Work out the finished part from the listing and answer in its coordinate system (mm). Face numbers are marked on the shaded views. A direction names the side the tool comes from. Coordinates: 2 decimals unless noted, no trailing zeros. Order: outer loops, then holes, each group sorted by start corner. A loop starts at its lowest first (then second) coordinate and runs counter-clockwise, first axis right, second up. Notation, with made-up numbers: M -21,19.5 L 17,19.5 A17 ccw 17,36.5 Z; hole C 62,43 d2. An arc over 180 degrees is marked long. Use a Markdown table: item, result.
from build123d import *

# Parameters (mm, degrees)
BOSS_EXTRUDE1_DEPTH     = 76.2
CHAMFER1_SIZE           = 16.51
CHAMFER2_SIZE           = 1
CUT_EXTRUDE1_DEPTH      = 3.425
SKETCH5_R               = 1.905
CUT_EXTRUDE2_DEPTH      = 114.174020707
CUT_EXTRUDE3_DEPTH      = 118.371627589
CUT_EXTRUDE3_DEPTH_BACK = 12.7
SKETCH6_R               = 6.35
SKETCH5_3_R             = 3.81
CUT_EXTRUDE4_DEPTH      = 12.7


with BuildPart() as part:
    # Sketch1 → Boss-Extrude1 (new body)
    with BuildSketch(Plane(origin=(0, 0, 0), x_dir=(1, 0, 0), z_dir=(0, 1, 0))):
        Polygon((-25.4, 47.146344636), (25.4, 47.146344636), (72.546344636, 0), (25.4, -47.146344636), (-25.4, -47.146344636), (-72.546344636, 0), align=None)
    extrude(amount=BOSS_EXTRUDE1_DEPTH)

    # SurfaceCut1
    split(bisect_by=Plane(origin=(0, 10.036699622, 10.036699622), x_dir=(-1, 0, 0), z_dir=(0, 0.7071067811865464, 0.7071067811865488)), keep=Keep.TOP)

    # SurfaceCut2
    split(bisect_by=Plane(origin=(0, 10.036699622, -10.036699622), x_dir=(1, 0, 0), z_dir=(0, 0.7071067811865464, -0.7071067811865488)), keep=Keep.TOP)

    # SurfaceCut3
    split(bisect_by=Plane(origin=(0, 50.8, 0), x_dir=(1, 0, 0), z_dir=(0, 1, 0)), keep=Keep.TOP)

    # Chamfer1
    chamfer1_edges = [part.edges().sort_by_distance(p)[0] for p in [
        (-57.183044257, 50.8, 15.363300378),
        (-57.183044257, 50.8, -15.363300378),
        (57.183044257, 50.8, 15.363300378),
        (57.183044257, 50.8, -15.363300378),
    ]]
    chamfer(chamfer1_edges, length=CHAMFER1_SIZE)

    # Chamfer2
    chamfer2_edges = [part.edges().sort_by_distance(p)[0] for p in [
        (72.546344636, 71.755, 0),
        (-72.546344636, 71.755, 0),
        (0, 76.2, 47.146344636),
        (48.973172318, 76.2, 23.573172318),
        (48.973172318, 76.2, -23.573172318),
        (0, 76.2, -47.146344636),
        (-48.973172318, 76.2, -23.573172318),
        (-48.973172318, 76.2, 23.573172318),
    ]]
    chamfer(chamfer2_edges, length=CHAMFER2_SIZE)

    # Sketch2 → Cut-Extrude1 (cut)
    with BuildSketch(Plane(origin=(0, 76.2, 0), x_dir=(1, 0, 0), z_dir=(0, 1, 0))):
        Polygon((-23.68275885, 45.681605271), (-69.36436412, 0), (-23.682753383, -45.681610738), align=None)
        Polygon((69.36436412, 0), (23.682756199, 45.681607921), (23.682745222, -45.681618898), align=None)
    extrude(amount=-CUT_EXTRUDE1_DEPTH, mode=Mode.SUBTRACT)

    # Sketch5 → Cut-Extrude2 (cut, through all)
    with BuildSketch(Plane(origin=(0, 10.036699622, -10.036699622), x_dir=(1, 0, 0), z_dir=(0, 0.7071067811865464, -0.7071067811865488))):
        with Locations(Location((0, -53.881536726, 0), (0, 0, 270))):
            Circle(SKETCH5_R)
    extrude(amount=CUT_EXTRUDE2_DEPTH, mode=Mode.SUBTRACT)

    # Sketch6 → Cut-Extrude3 (cut, two sides: drawn at the far end of the back side and taken through both)
    with BuildSketch(Plane(origin=(0, 36.977467985, -36.977467985), x_dir=(1, 0, 0), z_dir=(0, 0.7071067811865464, -0.7071067811865488)).offset(-CUT_EXTRUDE3_DEPTH_BACK)):
        with Locations(Location((0, -53.881536726, 0), (0, 0, 270))):
            Circle(SKETCH6_R)
    extrude(amount=CUT_EXTRUDE3_DEPTH + CUT_EXTRUDE3_DEPTH_BACK, mode=Mode.SUBTRACT)

    # Sketch5<3> → Cut-Extrude4 (cut)
    with BuildSketch(Plane(origin=(0, 10.036699622, -10.036699622), x_dir=(1, 0, 0), z_dir=(0, 0.7071067811865464, -0.7071067811865488))):
        with Locations(Location((0, -53.881536726, 0), (0, 0, 278.668745784))):
            Circle(SKETCH5_3_R)
    extrude(amount=CUT_EXTRUDE4_DEPTH, mode=Mode.SUBTRACT)


solid = part.part
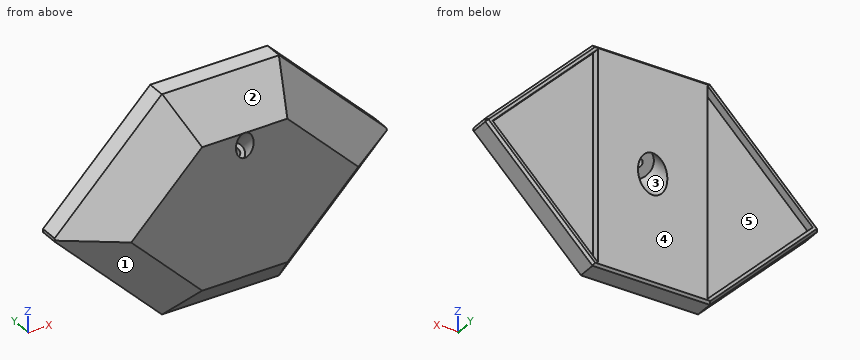
(1) Which of the six approach directions +Z, -Z, +X, -X, +Y, -Y give full straight-line access (tool end or side, diameter ignored) to the marked faces 4 and 5?
Conclusion:
| item | result |
|---|---|
| face 4 | +Z, -Z, +X, -X, +Y |
| face 5 | +Y |
(2) Straight lines are drawn through the part: L1, parallel to X at y = 73.75, z = 40.5; L2, parallel to X at y = 74.75, z = 0.5; L3, parallel to X at y = 74.75, z = 15. For each, find the intervals that lie inside material, in ascending order.
Conclusion:
| item | result |
|---|---|
| L1 | -32.05 to -28.86, -23.68 to 23.68, 28.86 to 32.05 |
| L2 | -71.84 to -68.86, -23.68 to -6.31, 6.31 to 23.68, 68.86 to 71.84 |
| L3 | -57.55 to -54.36, -23.68 to 23.68, 54.36 to 57.55 |
(3) Given P1, Ø3, axis at x = 28.5, z = 22, coming from the -Y side; P2, Ø2, axis at x = 43.5, y = 66, coming from the +Z side; P3, Ø4, axis at x = -32, y = 61, coming from the +Z side; P4, Ø13.5, axis at x = 37, z = 4.5, coming from the +Y side (3 decimals), each flat-ended and moving along its own axis, determine where each tip first touches the part or whether it passes through.
Conclusion:
| item | result |
|---|---|
| P1 | y = 50.8 |
| P2 | z = 28.93 |
| P3 | z = 35.09 |
| P4 | y = 72.775 |
(4) A cutting plane is placed at A-A (x = -15.5). Determine the outline of the cut face in (y, z).
Conclusion:
| item | result |
|---|---|
| outline | M 50.8,-30.73 L 67.22,-47.15 L 75.2,-47.15 L 76.2,-46.15 L 76.2,46.15 L 75.2,47.15 L 67.22,47.15 L 50.8,30.73 Z |
(5) A cutting plane is placed at D-D (x = 59). Determine the outline of the cut face in (y, z) (3 decimals).
Conclusion:
| item | result |
|---|---|
| outline | M 57.731,0 L 67.31,-13.546 L 75.2,-13.546 L 76.2,-12.132 L 76.2,-10.364 L 72.775,-10.364 L 72.775,10.364 L 76.2,10.364 L 76.2,12.132 L 75.2,13.546 L 67.31,13.546 Z |
(6) Determine the mould class of the marked faces 1, 2 and 3 for opening direction Z: pulls with the +Z half, pulls with the -Z half, needs draft (parallel to the pull), parting line crosses it, or undercut.
Conclusion:
| item | result |
|---|---|
| face 1 | pulls with the -Z half |
| face 2 | pulls with the +Z half |
| face 3 | undercut |
(7) A cutting plane is placed at C-C (y = 64.25). Give the number of separate pieces and of enclosed holes in the cut face, then the cut area to 3 significant figures.
Conclusion:
| item | result |
|---|---|
| separate pieces | 1 |
| enclosed holes | 2 |
| area | 8,090 mm2 |
(8) A cutting plane is placed at B-B (z = -20.5). Determine the outline of the cut face in (x, y) (3 decimals), then the cut area to 3 significant figures.
Conclusion:
| item | result |
|---|---|
| outline | M -52.046,67.31 L -28.698,50.8 L 28.698,50.8 L 52.046,67.31 L 52.046,75.2 L 50.632,76.2 L 48.864,76.2 L 48.864,72.775 L 23.683,72.775 L 23.683,76.2 L -23.683,76.2 L -23.683,72.775 L -48.864,72.775 L -48.864,76.2 L -50.632,76.2 L -52.046,75.2 Z |
| area | 2,080 mm2 |
